```python
from build123d import *

# Parameters (mm, degrees)
SKETCH1_W           = 139.7
SKETCH1_H           = 89
BOSS_EXTRUDE1_DEPTH = 5
SKETCH4_R           = 4.5
SKETCH4_R_2         = 2.5
BOSS_EXTRUDE2_DEPTH = 12
SKETCH12_R          = 2
CUT_EXTRUDE1_DEPTH  = 5
CUT_EXTRUDE2_START  = -10
SKETCH13_R          = 2.5
CUT_EXTRUDE2_DEPTH  = 10


with BuildPart() as part:
    # Sketch1 → Boss-Extrude1 (new body)
    with BuildSketch(Plane(origin=(0, 0, 0), x_dir=(1, 0, 0), z_dir=(0, 1, 0))):
        with Locations((-0.18185994, 0.363719879)):
            Rectangle(SKETCH1_W, SKETCH1_H)
    extrude(amount=BOSS_EXTRUDE1_DEPTH)

    # Sketch4 → Boss-Extrude2 (add)
    # profile 1 of 4: a face of its own
    with BuildSketch(Plane.XZ):
        with Locations(Location((-61.03185994, 28.136280121, 0), (0, 0, 270))):
            Circle(SKETCH4_R)
        with Locations(Location((-61.03185994, 28.136280121, 0), (0, 0, 270))):
            Circle(SKETCH4_R_2, mode=Mode.SUBTRACT)
    # profile 2 of 4: a face of its own
    with BuildSketch(Plane.XZ):
        with Locations(Location((49.66814006, 28.136280121, 0), (0, 0, 270))):
            Circle(SKETCH4_R)
        with Locations(Location((49.66814006, 28.136280121, 0), (0, 0, 270))):
            Circle(SKETCH4_R_2, mode=Mode.SUBTRACT)
    # profile 3 of 4: a face of its own
    with BuildSketch(Plane.XZ):
        with Locations(Location((-61.03185994, -25.363719879, 0), (0, 0, 270))):
            Circle(SKETCH4_R)
        with Locations(Location((-61.03185994, -25.363719879, 0), (0, 0, 270))):
            Circle(SKETCH4_R_2, mode=Mode.SUBTRACT)
    # profile 4 of 4: a face of its own
    with BuildSketch(Plane.XZ):
        with Locations(Location((49.66814006, -25.363719879, 0), (0, 0, 270))):
            Circle(SKETCH4_R)
        with Locations(Location((49.66814006, -25.363719879, 0), (0, 0, 270))):
            Circle(SKETCH4_R_2, mode=Mode.SUBTRACT)
    extrude(amount=BOSS_EXTRUDE2_DEPTH)

    # Sketch12 → Cut-Extrude1 (cut)
    with BuildSketch(Plane.XZ):
        with Locations(Location((-0.18185994, 24.136280121, 0), (0, 0, 270))):
            Circle(SKETCH12_R)
        with Locations(Location((-0.18185994, -24.863719879, 0), (0, 0, 270))):
            Circle(SKETCH12_R)
    extrude(amount=-CUT_EXTRUDE1_DEPTH, mode=Mode.SUBTRACT)

    # Sketch13 → Cut-Extrude2 (cut)
    with BuildSketch(Plane.XZ.offset(CUT_EXTRUDE2_START)):
        with Locations(Location((-61.03185994, 28.136280121, 0), (0, 0, 270))):
            Circle(SKETCH13_R)
        with Locations(Location((-61.03185994, -25.363719879, 0), (0, 0, 270))):
            Circle(SKETCH13_R)
        with Locations(Location((49.66814006, -25.363719879, 0), (0, 0, 270))):
            Circle(SKETCH13_R)
        with Locations(Location((49.66814006, 28.136280121, 0), (0, 0, 270))):
            Circle(SKETCH13_R)
    extrude(amount=CUT_EXTRUDE2_DEPTH, mode=Mode.SUBTRACT)


solid = part.part
```
The listing builds one solid part. Answer for the finished solid, in the listing's coordinates (mm). A direction names the side the tool comes from. Give positions to 0.01 mm unless a question says otherwise; leave off trailing zeros. Loops run counter-clockwise (first coordinate to the right, second up) from the corner with the lowest first, then second, coordinate; pieces in that order, holes last. Notation, with made-up numbers: (46, 26) - (88, 26) arc R18 ccw to (88, 60) - close; hole circle Ø8 at (-10.75, 11). An arc over 180 degrees is marked (long way). Answer as CSV lines item,"result". Start each with the question number.
Item 1: For faces 1 (the face through (-63.77, -5.916, -21.793)), 2 (the face through (-63, -12, 26)), determine the directions among +Z, -Z, +X, -X, +Y, -Y from which every point of the face is accessible in a straight line to the end or side of a thin tool.
Item 2: A cutting plane is placed at B-B on x = -13. Determine the outline of the cut face in (y, z), then the cut area to 3 significant figures.
Item 3: A cutting plane is placed at C-C on z = -37.5. Determine the outline of the cut face in (x, y).
Item 4: Find the intervals of material crossed by line 1 (X direction, y = -0.5, z = 28.5); line 2 (Z direction, x = 50, y = -5); line 3 (X direction, y = 3.75, z = 28.5), in increasing order. Write a range as from..to.
Item 5: The mould has two halves that part along Z. Classify faces 3 (the face through (45.275, -5.916, 29.112)), 4 (the face through (51.776, -3.381, 26.792)), 5 (the face through (69.668, 2, 0)), 6 (the face through (-1, 2, -44.864)): +Z half, -Z half, draft (parallel to the pull), parting line (faces both ways), or undercut.
Item 6: Each of these flat-tipped pins is pushed along its axis until it touches: pin 1 (2 mm diameter, centred on x = 31.5, z = 26.5, fed in from -Y); pin 2 (4 mm diameter, centred on y = -4, z = -27, fed in from -X); pin 3 (4.5 mm diameter, centred on x = -0.18, z = 24.14, fed in from +Y). Where does it stop, or does it pass through?
Item 7: A cutting plane is placed at A-A on y = -9.25. Determine the outline of the cut face in (x, z).
Found:
1,face 1,"-Y"
1,face 2,"+Z, -Z, +X, -X, -Y"
2,outline,"(0, -44.86) - (5, -44.86) - (5, 44.14) - (0, 44.14) - close"
2,area,"445 mm^2"
3,outline,"(-70.03, 0) - (69.67, 0) - (69.67, 5) - (-70.03, 5) - close"
4,line 1,"x = -65.52..-63.51, -58.56..-56.55, 45.18..47.19, 52.14..54.15"
4,line 2,"z = -29.85..-27.84, -22.89..-20.88, 23.65..25.66, 30.61..32.62"
4,line 3,"x = -70.03..-63.51, -58.56..47.19, 52.14..69.67"
5,face 3,"undercut"
5,face 4,"undercut"
5,face 5,"draft"
5,face 6,"-Z half"
6,pin 1,"stops at y = 0"
6,pin 2,"stops at x = -65.53"
6,pin 3,"stops at y = 5"
7,outline,"circle Ø9 at (-61.03, -25.36); circle Ø9 at (-61.03, 28.14); circle Ø9 at (49.67, -25.36); circle Ø9 at (49.67, 28.14); hole circle Ø5 at (-61.03, -25.36); hole circle Ø5 at (-61.03, 28.14); hole circle Ø5 at (49.67, -25.36); hole circle Ø5 at (49.67, 28.14)"
